Read the model definition and answer for the solid it produces. Units are mm, in the model's axes. A direction names the side the tool comes from. Coordinates: 2 decimals unless noted, no trailing zeros. Write each loop counter-clockwise with the first axis right and the second up, starting at its lowest first coordinate (ties: lowest second). Pieces come first, ordered by that corner, then holes. Notation, with made-up numbers: (75, 60.5) -> (114, 60.5) arc R29 ccw to (114, 88.5) -> close; hole circle Ø6 at (-12, 10). An arc over 180 degrees is marked (long way). Return JSON: item names as keys, results as strings.
from build123d import *

# Parameters (mm, degrees)
MODEL_R                 = 1.5
SALIENTE_EXTRUIR1_DEPTH = 1


with BuildPart() as part:
    # Model → Saliente-Extruir1 (new body)
    with BuildSketch(Plane.XY):
        with BuildLine():
            Line((6.261217919, 18.769360839), (-14.739513879, 9.794996238))
            ThreePointArc((-14.739513879, 9.794996238), (-18.828558612, 11.883464999), (-16.872209477, 16.037341099))
            Line((-16.872209477, 16.037341099), (6.261217919, 25.600360839))
            Line((6.261217919, 25.600360839), (39.261217919, 25.600360839))
            Line((39.261217919, 25.600360839), (39.261217919, 18.769360839))
            Line((39.261217919, 18.769360839), (6.261217919, 18.769360839))
        make_face()
        with Locations((33.761217919, 22.184860839)):
            Circle(MODEL_R, mode=Mode.SUBTRACT)
        with Locations((6.261217919, 22.184860839)):
            Circle(MODEL_R, mode=Mode.SUBTRACT)
        with Locations((-15.705782081, 12.950360839)):
            Circle(MODEL_R, mode=Mode.SUBTRACT)
    extrude(amount=SALIENTE_EXTRUIR1_DEPTH)


solid = part.part
1. For a pull along Y with two mould halves and no side action, classify faces 3 (the face through (39.261, 22.2, 0.5)), 4 (the face through (5.94, 20.72, 0.49)), 5 (the face through (-4.092, 14.345, 0.493)) as +Y half, -Y half, draft (parallel to the pull), parting line (faces both ways), or undercut.
Taken from the geometry:
{"face 3": "draft", "face 4": "undercut", "face 5": "-Y half"}
2. Consider L1, parallel to X at y = 21.25, z = 0.3; L2, parallel to X at y = 22.75, z = 0.3; L3, parallel to Y at x = 33.5, z = 0.45. Determine where each line is inside the solid, lowest interval first.
Taken from the geometry:
{"L1": "x = -4.26 to 5.09, 7.43 to 32.59, 34.93 to 39.26", "L2": "x = -0.63 to 4.87, 7.65 to 32.37, 35.15 to 39.26", "L3": "y = 18.77 to 20.71, 23.66 to 25.6"}
3. The part is cut by section A-A (y = 12.25). Determine the outline of the cut face in (x, z).
Taken from the geometry:
{"outline": "(-18.93, 0) -> (-17.03, 0) -> (-17.03, 1) -> (-18.93, 1) -> close; (-14.38, 0) -> (-8.99, 0) -> (-8.99, 1) -> (-14.38, 1) -> close"}
4. A flat-ended cylindrical pin translates along its axis: pin 1 Ø0.5 at (x, z) = (29.5, 0.5) entering from -Y. Find the tip coordinate at first contact, or state that the pin passes through.
Taken from the geometry:
{"pin 1": "stops at y = 18.77"}
5. The part is cut by section D-D (y = 15.5). Determine the outline of the cut face in (x, z), then the cut area to 3 significant figures.
Taken from the geometry:
{"outline": "(-17.8, 0) -> (-1.39, 0) -> (-1.39, 1) -> (-17.8, 1) -> close", "area": "16.4 mm2"}
6. The part is cut by section C-C (x = 10). Determine the outline of the cut face in (y, z).
Taken from the geometry:
{"outline": "(18.77, 0) -> (25.6, 0) -> (25.6, 1) -> (18.77, 1) -> close"}
7. The part is cut by section B-B (z = 0.3). Determine the outline of the cut face in (x, y) (3 decimals), then the cut area to 3 significant figures.
Taken from the geometry:
{"outline": "(-16.872, 16.037) arc R3.3 ccw to (-14.74, 9.795) -> (6.261, 18.769) -> (39.261, 18.769) -> (39.261, 25.6) -> (6.261, 25.6) -> close; hole circle Ø3 at (-15.706, 12.95); hole circle Ø3 at (6.261, 22.185); hole circle Ø3 at (33.761, 22.185)", "area": "375 mm2"}
8. A tool of negligible diameter and unlimited length cuts with its end or side. For faces 1 (the face through (23, 18.769, 0.5)), 2 (the face through (22.5, 25.6, 0.5)), from which of +Z, -Z, +X, -X, +Y, -Y can it reach the whole face along a straight path? Write none if from no direction.
Taken from the geometry:
{"face 1": "+Z, -Z, +X, -Y", "face 2": "+Z, -Z, +X, -X, +Y"}
